```python
from build123d import *

# Parameters (mm, degrees)
SKETCH1_W            = 192
SKETCH1_H            = 96
BOSS_EXTRUDE1_DEPTH  = 3
M3_CLEARANCE_HOLE1_D = 3.4
SKETCH6_W            = 15
SKETCH6_H            = 40
SKETCH6_W_2          = 20
SKETCH6_H_2          = 15
CUT_EXTRUDE1_DEPTH   = 215.683487954
M3_CLEARANCE_HOLE2_D = 3.4


with BuildPart() as part:
    # Sketch1 → Boss-Extrude1 (new body)
    with BuildSketch(Plane(origin=(0, 0, 0), x_dir=(1, 0, 0), z_dir=(0, 1, 0))):
        with Locations((96, 48)):
            Rectangle(SKETCH1_W, SKETCH1_H)
    extrude(amount=BOSS_EXTRUDE1_DEPTH)

    # M3 Clearance Hole1 (through all)
    with Locations(Plane(origin=(0, 0, 0), x_dir=(-1, 0, 0), z_dir=(0, -1, 0))):
        with Locations((-13, 9.1), (-179, 9.1), (-179, 86.9), (-13, 86.9)):
            Hole(M3_CLEARANCE_HOLE1_D / 2)

    # Sketch6 → Cut-Extrude1 (cut, through all)
    with BuildSketch(Plane.XZ):
        with Locations((19.8, -48)):
            Rectangle(SKETCH6_W, SKETCH6_H)
        with Locations((172.2, -48)):
            Rectangle(SKETCH6_W, SKETCH6_H)
        with Locations((113, -44)):
            Rectangle(SKETCH6_W_2, SKETCH6_H_2)
    extrude(amount=-CUT_EXTRUDE1_DEPTH, mode=Mode.SUBTRACT)

    # M3 Clearance Hole2 (through all)
    with Locations(Plane(origin=(0, 0, 0), x_dir=(-1, 0, 0), z_dir=(0, -1, 0))):
        with Locations((-33, 58.4), (-33, 30.5), (-85.11, 25.4), (-83.8, 73.6)):
            Hole(M3_CLEARANCE_HOLE2_D / 2)


solid = part.part
```
Input: part model. Units: mm. Frame: model coordinates. Coordinates: 2 decimals unless noted, no trailing zeros. Loops run counter-clockwise (first coordinate to the right, second up) from the corner with the lowest first, then second, coordinate; pieces in that order, holes last. Notation, with made-up numbers: M 4.25,4 L 24.25,4 A36 cw 24.25,38 Z; hole C 31.5,-38 d6. An arc over 180 degrees is marked long. Answer in a Markdown table with one row per item.
1. Section C-C, the plane z = -38.5. Output: boundary loops of the cut face in (x, y), then the cut area to 3 significant figures.
Response:
| item | result |
|---|---|
| outline | M 0,0 L 12.3,0 L 12.3,3 L 0,3 Z; M 27.3,0 L 103,0 L 103,3 L 27.3,3 Z; M 123,0 L 164.7,0 L 164.7,3 L 123,3 Z; M 179.7,0 L 192,0 L 192,3 L 179.7,3 Z |
| area | 426 mm2 |
2. Material intervals for line 1 (X direction, y = 2, z = -60.5); line 2 (X direction, y = 1.2, z = -38.5); line 3 (X direction, y = 1.9, z = -9.1), sorted ascending.
Response:
| item | result |
|---|---|
| line 1 | x = 0 to 12.3, 27.3 to 164.7, 179.7 to 192 |
| line 2 | x = 0 to 12.3, 27.3 to 103, 123 to 164.7, 179.7 to 192 |
| line 3 | x = 0 to 11.3, 14.7 to 177.3, 180.7 to 192 |
3. Draft query along X for faces 1 (the cylindrical face through (180.57, 1.52, -8.45)), 2 (the flat face through (95, 3, -49)). Return one class per face: pulls with the +X half, pulls with the -X half, needs draft (parallel to the pull), parting line crosses it, or undercut.
Response:
| item | result |
|---|---|
| face 1 | undercut |
| face 2 | needs draft |
4. Section B-B, the plane y = 1.75. Count the separate pieces of the cut face and the enclosed holes in it, then the cut area to 3 significant figures.
Response:
| item | result |
|---|---|
| separate pieces | 1 |
| enclosed holes | 11 |
| area | 16,900 mm2 |
5. Section A-A, the plane z = -65. Output: boundary loops of the cut face in (x, y).
Response:
| item | result |
|---|---|
| outline | M 0,0 L 12.3,0 L 12.3,3 L 0,3 Z; M 27.3,0 L 164.7,0 L 164.7,3 L 27.3,3 Z; M 179.7,0 L 192,0 L 192,3 L 179.7,3 Z |
6. First-contact query: pin 1 (2.5 mm diameter, centred on x = 179, z = -9.1, fed in from -Y). Flat tip, straight axial feed; report the tip coordinate or a pass-through.
Response:
| item | result |
|---|---|
| pin 1 | passes through |
